from build123d import *

# Parameters (mm, degrees)
EXTRUDE_1_DEPTH                 = 10
SKETCH_4_W                      = 7.875
SKETCH_4_H                      = 20
EXTRUDE_2_DEPTH                 = 40
CUT_EXTRUDE_1_REACH             = 116.35
SKETCH_5_R                      = 2.2
CUT_EXTRUDE_1_DIRECTION_2_DEPTH = 53
CUT_EXTRUDE_2_REACH             = 107.272
SKETCH_6_R                      = 2.15
FILLET_1_R                      = 5
FILLET_2_R                      = 5
SKETCH_7_W                      = 7.875
SKETCH_7_H                      = 20
EXTRUDE_3_DEPTH                 = 18
CUT_EXTRUDE_3_REACH             = 116.35
SKETCH_8_R                      = 2.2
EXTRUDE_8_DEPTH                 = 20
SKETCH_15_W                     = 52.625
SKETCH_15_H                     = 20
EXTRUDE_9_DEPTH                 = 40
CUT_EXTRUDE_START               = -7.875
SKETCH_14_R                     = 4.5
CUT_EXTRUDE_8_DEPTH             = 54
CUT_EXTRUDE_10_DEPTH            = 20
EXTRUDE_10_DEPTH                = 10
EXTRUDE_11_DEPTH                = 17.5
CUT_EXTRUDE_11_DEPTH            = 64


with BuildPart() as part:
    # 草图1 → 凸台-拉伸1 (new body)
    with BuildSketch(Plane(origin=(0, 0, 0), x_dir=(1, 0, 0), z_dir=(0, 1, 0))):
        Polygon((5.931150433, 81.572237736), (53.180774799, 81.572237736), (53.180774799, 61.572237736), (42.680774799, 42.721022935), (42.680774799, 31.757290204), (42.680774799, -57.600660719), (42.680774799, -67.427762264), (0.431150433, -67.427762264), (-17.319225201, -67.427762264), (-17.319225201, 81.572237736), align=None)
        Polygon((47.930774799, 61.572237736), (42.680774799, 61.572237736), (42.680774799, 52.689495612), align=None, mode=Mode.SUBTRACT)
        Polygon((25.906315323, 61.572237736), (-7.319225201, 61.572237736), (-7.319225201, -49.220735683), align=None, mode=Mode.SUBTRACT)
        Polygon((0.431150433, -52.427762264), (32.680774799, -52.427762264), (32.680774799, 56.508121895), align=None, mode=Mode.SUBTRACT)
    extrude(amount=EXTRUDE_1_DEPTH)

    # 草图4 → 凸台-拉伸2 (add)
    with BuildSketch(Plane(origin=(0, 10, 0), x_dir=(1, 0, 0), z_dir=(0, 1, 0))):
        with Locations((49.243274799, 71.572237736)):
            Rectangle(SKETCH_4_W, SKETCH_4_H)
    extrude(amount=EXTRUDE_2_DEPTH)

    # 草图5 → 切除-拉伸1 (cut, up to next)
    with BuildSketch(Plane.ZY.offset(-45.305774799), mode=Mode.PRIVATE) as cut_extrude_1_sk1:
        with Locations(Location((-71.572237736, 14.7, 0), (0, 0, 180))):
            Circle(SKETCH_5_R)
    cut_extrude_1_tool1 = extrude(cut_extrude_1_sk1.sketch, amount=-CUT_EXTRUDE_1_REACH, mode=Mode.PRIVATE) & part.part
    # 草图5 → 切除-拉伸1 (cut, up to next)
    with BuildSketch(Plane.ZY.offset(-45.305774799), mode=Mode.PRIVATE) as cut_extrude_1_sk2:
        with Locations(Location((-71.572237736, 40.7, 0), (0, 0, 180))):
            Circle(SKETCH_5_R)
    cut_extrude_1_tool2 = extrude(cut_extrude_1_sk2.sketch, amount=-CUT_EXTRUDE_1_REACH, mode=Mode.PRIVATE) & part.part
    add(cut_extrude_1_tool1.solids().sort_by_distance((45.305775, 14.7, -71.572238))[0], mode=Mode.SUBTRACT)
    add(cut_extrude_1_tool2.solids().sort_by_distance((45.305775, 40.7, -71.572238))[0], mode=Mode.SUBTRACT)

    # 草图5 → 切除-拉伸1 direction 2 (cut)
    with BuildSketch(Plane.ZY.offset(-45.305774799)):
        with Locations(Location((-71.572237736, 14.7, 0), (0, 0, 180))):
            Circle(SKETCH_5_R)
        with Locations(Location((-71.572237736, 40.7, 0), (0, 0, 180))):
            Circle(SKETCH_5_R)
    extrude(amount=CUT_EXTRUDE_1_DIRECTION_2_DEPTH, mode=Mode.SUBTRACT)

    # 草图6 → 切除-拉伸2 (cut, up to next)
    with BuildSketch(Plane(origin=(0, 10, 0), x_dir=(1, 0, 0), z_dir=(0, 1, 0)), mode=Mode.PRIVATE) as cut_extrude_2_sk1:
        with Locations(Location((-8.019225201, -61.542634482, 0), (0, 0, 270))):
            Circle(SKETCH_6_R)
    cut_extrude_2_tool1 = extrude(cut_extrude_2_sk1.sketch, amount=-CUT_EXTRUDE_2_REACH, mode=Mode.PRIVATE) & part.part
    # 草图6 → 切除-拉伸2 (cut, up to next)
    with BuildSketch(Plane(origin=(0, 10, 0), x_dir=(1, 0, 0), z_dir=(0, 1, 0)), mode=Mode.PRIVATE) as cut_extrude_2_sk2:
        with Locations(Location((32.680774799, -58.692634482, 0), (0, 0, 270))):
            Circle(SKETCH_6_R)
    cut_extrude_2_tool2 = extrude(cut_extrude_2_sk2.sketch, amount=-CUT_EXTRUDE_2_REACH, mode=Mode.PRIVATE) & part.part
    add(cut_extrude_2_tool1.solids().sort_by_distance((-8.019225, 10, 61.542634))[0], mode=Mode.SUBTRACT)
    add(cut_extrude_2_tool2.solids().sort_by_distance((32.680775, 10, 58.692634))[0], mode=Mode.SUBTRACT)

    # 圆角1
    fillet_1_edges = [part.edges().sort_by_distance(p)[0] for p in [
        (-17.319225201, 5, 67.427762264),
        (-17.319225201, 5, -81.572237736),
        (42.680774799, 5, 67.427762264),
    ]]
    fillet(fillet_1_edges, radius=FILLET_1_R)

    # 圆角2
    fillet_2_edges = [part.edges().sort_by_distance(p)[0] for p in [
        (32.680774799, 5, 52.427762264),
    ]]
    fillet(fillet_2_edges, radius=FILLET_2_R)

    # 草图7 → 凸台-拉伸3 (add)
    with BuildSketch(Plane.XZ):
        with Locations((49.243274799, -71.572237736)):
            Rectangle(SKETCH_7_W, SKETCH_7_H)
    extrude(amount=EXTRUDE_3_DEPTH)

    # 草图8 → 切除-拉伸3 (cut, up to next)
    with BuildSketch(Plane.ZY.offset(-45.305774799), mode=Mode.PRIVATE) as cut_extrude_3_sk1:
        with Locations((-71.572237736, -11.3)):
            Circle(SKETCH_8_R)
    cut_extrude_3_tool1 = extrude(cut_extrude_3_sk1.sketch, amount=-CUT_EXTRUDE_3_REACH, mode=Mode.PRIVATE) & part.part
    add(cut_extrude_3_tool1.solids().sort_by_distance((45.305775, -11.3, -71.572238))[0], mode=Mode.SUBTRACT)

    # 草图13 → 凸台-拉伸8 (add)
    with BuildSketch(Plane.XY.offset(-61.572237736)):
        Polygon((45.305774799, 0), (45.305774799, -18), (-7.319225201, 0), align=None)
    extrude(amount=-EXTRUDE_8_DEPTH)

    # 草图15 → 凸台-拉伸9 (add)
    with BuildSketch(Plane(origin=(0, 10, 0), x_dir=(1, 0, 0), z_dir=(0, 1, 0))):
        with Locations((18.993274799, 71.572237736)):
            Rectangle(SKETCH_15_W, SKETCH_15_H)
    extrude(amount=EXTRUDE_9_DEPTH)

    # 草图14 → 切除-拉伸8 (cut)
    with BuildSketch(Plane(origin=(53.180774799, 0, 0), x_dir=(0, 0, -1), z_dir=(1, 0, 0)).offset(CUT_EXTRUDE_START)):
        with Locations((71.572237736, 40.7)):
            Circle(SKETCH_14_R)
        with Locations((71.572237736, 14.7)):
            Circle(SKETCH_14_R)
        with Locations((71.572237736, -11.3)):
            Circle(SKETCH_14_R)
    extrude(amount=-CUT_EXTRUDE_8_DEPTH, mode=Mode.SUBTRACT)

    # 草图17 → 切除-拉伸10 (cut)
    with BuildSketch(Plane.XY.offset(-61.572237736)):
        Polygon((-7.319225201, 10), (-7.319225201, 50), (45.305774799, 50), align=None)
    extrude(amount=-CUT_EXTRUDE_10_DEPTH, mode=Mode.SUBTRACT)

    # 草图18 → 凸台-拉伸10 (add)
    with BuildSketch(Plane(origin=(0, 10, 0), x_dir=(1, 0, 0), z_dir=(0, 1, 0))):
        Polygon((-7.319225201, 32.572237736), (17.209548321, 32.572237736), (20.208433494, 42.572237736), (-7.319225201, 42.572237736), align=None)
        Polygon((25.594741772, 32.572237736), (32.680774799, 32.572237736), (32.680774799, 56.508121895), align=None)
        Polygon((42.680774799, 61.572237736), (42.680774799, 52.689495612), (47.930774799, 61.572237736), align=None)
    extrude(amount=-EXTRUDE_10_DEPTH)

    # 草图19 → 凸台-拉伸11 (add)
    with BuildSketch(Plane.XZ):
        Polygon((-17.319225201, -32.572237736), (-17.319225201, -42.572237736), (42.680774799, -42.721022935), (42.680774799, -32.572237736), align=None)
    extrude(amount=EXTRUDE_11_DEPTH)

    # 草图20 → 切除-拉伸11 (cut)
    with BuildSketch(Plane.ZY.offset(17.319225201)):
        Polygon((-42.572237736, -17.5), (-32.572237736, -17.5), (-32.572237736, -16.5), align=None)
    extrude(amount=-CUT_EXTRUDE_11_DEPTH, mode=Mode.SUBTRACT)


solid = part.part
Part model, mm, in its own coordinate system. A direction names the side the tool comes from. Coordinates: 2 decimals unless noted, no trailing zeros. Loops run counter-clockwise (first coordinate to the right, second up) from the corner with the lowest first, then second, coordinate; pieces in that order, holes last. Notation, with made-up numbers: (-39.75, 29.5) -> (-15.75, 29.5) arc R33 ccw to (-15.75, 57.5) -> close; hole circle Ø1 at (46.5, 6). An arc over 180 degrees is marked (long way). Use a Markdown table: item, result. Add a question column.
Item 1: Probe probe 1 along Z at (x, y) = (25, -11); probe 2 along Y at (x, z) = (38, -47.5); probe 3 along Z at (x, y) = (38, 5). List the from-to ranges inside material, lowest first.
Item 2: Which spindle directions (+Z, -Z, +X, -X, +Y, -Y) get a long thin tool onto all of the face, cutting with end or side? Do faces 4 (the flat face through (29, 16, -61.572)), 5 (the flat face through (42.681, 3, -3)), 6 (the flat face through (45.306, -10, -74)), 7 (the flat face through (36, 0, -52)). Say none if no direction does.
Item 3: Flat gauge pins, fed straight in: P1, Ø4, axis at x = 31.5, z = -13.5, coming from the +Y side; P2, Ø4, axis at x = -8.02, z = 61.54, coming from the -Y side; P3, Ø8, axis at y = -11.3, z = -71.57, coming from the -X side; P4, Ø3, axis at y = 3.5, z = -1.5, coming from the +X side. Where does each tip first touch, or does it go through?
Item 4: Band-saw the part on B-B on y = 40.7. Write the cut outline in (x, z), plus the area to 3 significant figures.
Item 5: Band-saw the part on D-D on z = -50. Write the cut outline in (x, y), plus the area to 3 significant figures.
Item 6: Band-saw the part on C-C on x = 3.5. Write the cut outline in (y, z), plus the area to 3 significant figures.
Item 7: Band-saw the part on A-A on z = 16. Write the cut outline in (x, y).
Item 8: Pull direction X, two halves, no side cores. Call faces 1 (the flat face through (-12, 0, -62)), 2 (the flat face through (19.362, -9.126, -66.988)), 3 (the cylindrical face through (30.58, 5.07, 58.23)): +X half, -X half, draft (parallel to the pull), parting line (faces both ways), or undercut.
Geometry says:
| question | item | result |
|---|---|---|
| 1 | probe 1 | -81.57 to -76.06, -67.08 to -61.57, -42.68 to -32.57 |
| 1 | probe 2 | 0 to 10 |
| 1 | probe 3 | -81.57 to 67.42 |
| 2 | face 4 | none |
| 2 | face 5 | +Z, +X, +Y, -Y |
| 2 | face 6 | -X |
| 2 | face 7 | +X, -X, -Y |
| 3 | P1 | y = 10 |
| 3 | P2 | through |
| 3 | P3 | x = 45.31 |
| 3 | P4 | x = 42.68 |
| 4 | outline | (33.07, -81.57) -> (53.18, -81.57) -> (53.18, -73.77) -> (45.31, -73.77) -> (45.31, -76.07) -> (33.07, -76.07) -> close; (33.07, -67.07) -> (45.31, -67.07) -> (45.31, -69.37) -> (53.18, -69.37) -> (53.18, -61.57) -> (33.07, -61.57) -> close |
| 4 | area | 257 mm² |
| 5 | outline | (-17.32, 0) -> (-7.32, 0) -> (-7.32, 10) -> (-17.32, 10) -> close; (22.44, 0) -> (46.74, 0) -> (46.74, 10) -> (22.44, 10) -> close |
| 5 | area | 343 mm² |
| 6 | outline | (-17.5, -42.62) -> (0, -42.62) -> (0, -42.57) -> (10, -42.57) -> (10, -32.57) -> (-16.5, -32.57) -> (-17.5, -42.57) -> close; (-3.7, -81.57) -> (18.22, -81.57) -> (18.22, -74.37) arc R4.5 cw (long way) to (18.22, -68.77) -> (18.22, -61.57) -> (-3.7, -61.57) -> close; (0, 13.14) -> (10, 13.14) -> (10, 42.06) -> (0, 42.06) -> close; (0, 52.43) -> (10, 52.43) -> (10, 67.43) -> (0, 67.43) -> close |
| 6 | area | 1,090 mm² |
| 7 | outline | (-17.32, 0) -> (-7.32, 0) -> (-7.32, 10) -> (-17.32, 10) -> close; (2.64, 0) -> (11.22, 0) -> (11.22, 10) -> (2.64, 10) -> close; (32.68, 0) -> (42.68, 0) -> (42.68, 10) -> (32.68, 10) -> close |
| 8 | face 1 | draft |
| 8 | face 2 | -X half |
| 8 | face 3 | undercut |
